```python
from build123d import *

# Parameters (mm, degrees)
SKETCH1_W           = 26.67
SKETCH1_H           = 26.67
BOSS_EXTRUDE1_DEPTH = 5.08
SKETCH9_W           = 41.91
SKETCH9_H           = 41.91
BOSS_EXTRUDE7_DEPTH = 203.2
CUT_EXTRUDE4_DEPTH  = 42.91
SKETCH11_R          = 3.175
CUT_EXTRUDE5_DEPTH  = 42.91
SKETCH12_W          = 41.91
SKETCH12_H          = 25.4
BOSS_EXTRUDE8_DEPTH = 25.4
SKETCH13_R          = 3.175
CUT_EXTRUDE6_DEPTH  = 26.4
FILLET2_R           = 3.81
FILLET3_R           = 7.62


with BuildPart() as part:
    # Sketch1 → Boss-Extrude1 (new body)
    with BuildSketch(Plane(origin=(0, 0, 0), x_dir=(1, 0, 0), z_dir=(0, 1, 0))):
        Rectangle(SKETCH1_W, SKETCH1_H)
    extrude(amount=BOSS_EXTRUDE1_DEPTH)

    # Sketch9 → Boss-Extrude7 (add)
    with BuildSketch(Plane.XZ):
        Rectangle(SKETCH9_W, SKETCH9_H)
    extrude(amount=-BOSS_EXTRUDE7_DEPTH)

    # Sketch10 → Cut-Extrude4 (cut, through all)
    with BuildSketch(Plane.XY.offset(20.955)):
        with BuildLine():
            Line((-13.335, 185.42), (-13.335, 203.2))
            Line((-13.335, 203.2), (13.335, 203.2))
            Line((13.335, 203.2), (13.335, 185.42))
            ThreePointArc((13.335, 185.42), (11.103153673, 180.031846327), (5.715, 177.8))
            Line((5.715, 177.8), (-5.715, 177.8))
            ThreePointArc((-5.715, 177.8), (-11.103153673, 180.031846327), (-13.335, 185.42))
        make_face()
    extrude(amount=-CUT_EXTRUDE4_DEPTH, mode=Mode.SUBTRACT)

    # Sketch11 → Cut-Extrude5 (cut, through all)
    with BuildSketch(Plane.ZY.offset(20.955)):
        with Locations((-9.525, 195.58)):
            Circle(SKETCH11_R)
        with Locations((9.525, 195.58)):
            Circle(SKETCH11_R)
    extrude(amount=-CUT_EXTRUDE5_DEPTH, mode=Mode.SUBTRACT)

    # Sketch12 → Boss-Extrude8 (add)
    with BuildSketch(Plane.XY.offset(20.955)):
        with Locations((0, 12.7)):
            Rectangle(SKETCH12_W, SKETCH12_H)
    boss_extrude8 = extrude(amount=BOSS_EXTRUDE8_DEPTH)

    # Sketch13 → Cut-Extrude6 (cut, through all)
    with BuildSketch(Plane(origin=(0, 25.4, 0), x_dir=(1, 0, 0), z_dir=(0, 1, 0))):
        with Locations((-9.525, -29.845)):
            Circle(SKETCH13_R)
        with Locations((9.525, -29.845)):
            Circle(SKETCH13_R)
    cut_extrude6 = extrude(amount=-CUT_EXTRUDE6_DEPTH, mode=Mode.SUBTRACT)

    # Mirror1: Boss-Extrude8, Cut-Extrude6 across plane
    add(boss_extrude8.mirror(Plane.XY))
    add(cut_extrude6.mirror(Plane.XY), mode=Mode.SUBTRACT)

    # Fillet2
    fillet2_edges = [part.edges().sort_by_distance(p)[0] for p in [
        (20.955, 114.3, -20.955),
        (-20.955, 114.3, -20.955),
        (-20.955, 114.3, 20.955),
        (20.955, 114.3, 20.955),
    ]]
    fillet(fillet2_edges, radius=FILLET2_R)

    # Fillet3
    fillet3_edges = [part.edges().sort_by_distance(p)[0] for p in [
        (0, 0, 46.355),
        (0, 25.4, 46.355),
        (0, 25.4, -46.355),
        (0, 0, -46.355),
    ]]
    fillet(fillet3_edges, radius=FILLET3_R)


solid = part.part
```
Verification items for the finished model (mm, model axes). A direction names the side the tool comes from. Coordinates: 2 decimals unless noted, no trailing zeros. Loops run counter-clockwise (first coordinate to the right, second up) from the corner with the lowest first, then second, coordinate; pieces in that order, holes last. Notation, with made-up numbers: (-40, 30) - (-6, 30) arc R19 cw to (-6, 52) - close; hole circle Ø4 at (-5, 20.5). An arc over 180 degrees is marked (long way). Return JSON: item names as keys, results as strings.
1. Section check A-A, the plane y = 195.58. Record the boundary of the cut face in (x, z) (3 decimals), then the cut area to 3 significant figures.
Established:
{"outline": "(-20.955, -17.145) arc R3.81 ccw to (-17.145, -20.955) - (-13.335, -20.955) - (-13.335, -12.7) - (-20.955, -12.7) - close; (-20.955, -6.35) - (-13.335, -6.35) - (-13.335, 6.35) - (-20.955, 6.35) - close; (-20.955, 12.7) - (-13.335, 12.7) - (-13.335, 20.955) - (-17.145, 20.955) arc R3.81 ccw to (-20.955, 17.145) - close; (13.335, -20.955) - (17.145, -20.955) arc R3.81 ccw to (20.955, -17.145) - (20.955, -12.7) - (13.335, -12.7) - close; (13.335, -6.35) - (20.955, -6.35) - (20.955, 6.35) - (13.335, 6.35) - close; (13.335, 12.7) - (20.955, 12.7) - (20.955, 17.145) arc R3.81 ccw to (17.145, 20.955) - (13.335, 20.955) - close", "area": "433 mm2"}
2. Thickness scan on L1, parallel to Z at x = 16.75, y = 195.58 (3 decimals); L2, parallel to Y at x = -15, z = 9.5; L3, parallel to X at y = 190, z = 14 (3 decimals). Record the ranges inside material, lowest first.
Established:
{"L1": "z = -20.955 to -12.7, -6.35 to 6.35, 12.7 to 20.955", "L2": "y = 0 to 192.41, 198.75 to 203.2", "L3": "x = -20.955 to -13.335, 13.335 to 20.955"}
3. Tool access check on faces 4 (the flat face through (0, 113, 20.955)), 5 (the cylindrical face through (-19.87, 115.54, 19.81)), 6 (the cylindrical face through (-19.87, 115.54, -19.81)). Record the directions out of +Z, -Z, +X, -X, +Y, -Y that give a thin tool (end or side, any length) a straight path to the whole face; none if there is none.
Established:
{"face 4": "+Z, +X, -X, +Y", "face 5": "+Z, -X, +Y", "face 6": "-Z, -X, +Y"}
4. Section check C-C, the plane y = 71. Record the boundary of the cut face in (x, z) (3 decimals), then the cut area to 3 significant figures.
Established:
{"outline": "(-20.955, -17.145) arc R3.81 ccw to (-17.145, -20.955) - (17.145, -20.955) arc R3.81 ccw to (20.955, -17.145) - (20.955, 17.145) arc R3.81 ccw to (17.145, 20.955) - (-17.145, 20.955) arc R3.81 ccw to (-20.955, 17.145) - close", "area": "1,740 mm2"}
5. Go/stop test with flat-tipped pins: pin 1 (4 mm diameter, centred on x = 0, y = 86, fed in from -Z) (3 decimals); pin 2 (17.5 mm diameter, centred on x = 0.5, z = -33, fed in from +Y); pin 3 (3.5 mm diameter, centred on x = -0.5, z = 10, fed in from +Y). Record where each tip stops, or that it passes through.
Established:
{"pin 1": "stops at z = -20.955", "pin 2": "stops at y = 25.4", "pin 3": "stops at y = 177.8"}
6. Section check B-B, the plane z = -10. Record the boundary of the cut face in (x, y) (3 decimals).
Established:
{"outline": "(-20.955, 0) - (20.955, 0) - (20.955, 192.441) - (13.335, 192.441) - (13.335, 185.42) arc R7.62 cw to (5.715, 177.8) - (-5.715, 177.8) arc R7.62 cw to (-13.335, 185.42) - (-13.335, 192.441) - (-20.955, 192.441) - close; (-20.955, 198.719) - (-13.335, 198.719) - (-13.335, 203.2) - (-20.955, 203.2) - close; (13.335, 198.719) - (20.955, 198.719) - (20.955, 203.2) - (13.335, 203.2) - close"}
7. Mould release check, pull along Y, two halves, no side actions. Record for faces 1 (the flat face through (0, 13, 46.355)), 2 (the cylindrical face through (17.09, 192.48, -10.21)), 3 (the cylindrical face through (-11.04, 179.97, 0.29)): +Y half, -Y half, draft (parallel to the pull), parting line (faces both ways), or undercut.
Established:
{"face 1": "draft", "face 2": "undercut", "face 3": "+Y half"}
8. Section check D-D, the plane x = -10. Record the boundary of the cut face in (y, z) (3 decimals).
Established:
{"outline": "(0, -38.735) arc R7.62 ccw to (7.62, -46.355) - (17.78, -46.355) arc R7.62 ccw to (25.4, -38.735) - (25.4, -32.984) - (0, -32.984) - close; (0, -26.706) - (25.4, -26.706) - (25.4, -20.955) - (179.119, -20.955) - (179.119, 20.955) - (25.4, 20.955) - (25.4, 26.706) - (0, 26.706) - close; (0, 32.984) - (25.4, 32.984) - (25.4, 38.735) arc R7.62 ccw to (17.78, 46.355) - (7.62, 46.355) arc R7.62 ccw to (0, 38.735) - close"}
